Here's how the part is built. I have some questions about the finished solid (model axes, mm). Give positions to 0.01 mm unless a question says otherwise; leave off trailing zeros. Write each loop counter-clockwise with the first axis right and the second up, starting at its lowest first coordinate (ties: lowest second). Pieces come first, ordered by that corner, then holes. Notation, with made-up numbers: (-10.75, -7.5) - (10.25, -7.5) arc R20 cw to (10.25, 18.5) - close; hole circle Ø7 at (36, -18.5). An arc over 180 degrees is marked (long way). Use a Markdown table: item, result.
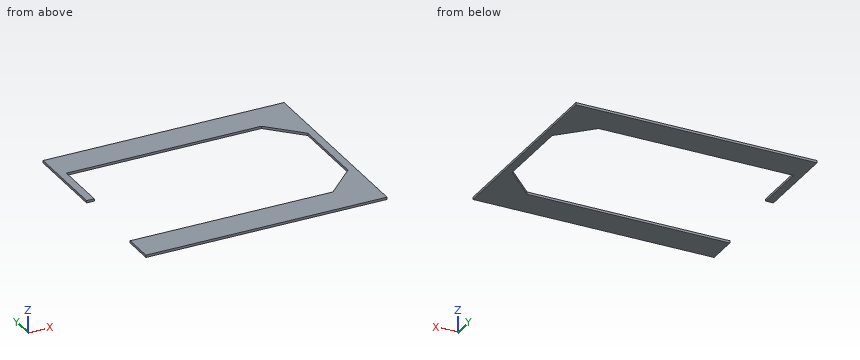
Autodesk Inventor part; units mm, degrees
ref_plane "YZ Plane" through (0, 0, 0) normal (1, 0, 0) x (0, 1, 0)
ref_plane "XZ Plane" through (0, 0, 0) normal (0, 1, 0) x (-1, 0, 0)
ref_plane "XY Plane" through (0, 0, 0) normal (0, 0, 1) x (1, 0, 0)
sketch "Эскиз1" plane through (0, 0, 0) normal (0, 0, 1) x (1, 0, 0)
  line L0 (0, 0) -> (-80.25, 0) construction
  line L1 (-80.25, 0) -> (-80.25, -18.086) construction
  line L2 (-80.25, -18.086) -> (0, -18.086) construction
  line L3 (0, -18.086) -> (0, 0) construction
  line L4 (-80.25, -18.086) -> (-80.25, -40.587) construction
  line L5 (-80.25, -18.086) -> (-57.749, -18.086) construction
  line L6 (-80.25, -40.587) -> (76.75, -40.587)
  line L7 (76.75, -40.587) -> (76.75, 90.413)
  line L8 (76.75, 90.413) -> (-80.25, 90.413)
  line L9 (-80.25, 90.413) -> (-80.25, -40.587)
  line L10 (-80.25, -40.587) -> (76.75, -40.587)
  line L11 (76.75, -40.587) -> (76.75, -20.587)
  line L12 (76.75, -20.587) -> (-80.25, -20.587)
  line L13 (-80.25, -20.587) -> (-80.25, -40.587)
  line L14 (76.75, 90.413) -> (-80.25, 90.413)
  line L15 (-80.25, 90.413) -> (-80.25, 70.413)
  line L16 (-80.25, 70.413) -> (76.75, 70.413)
  line L17 (76.75, 70.413) -> (76.75, 90.413)
  line L18 (-80.25, -40.587) -> (-75.25, -40.587)
  line L19 (-75.25, -40.587) -> (-75.25, 90.413)
  line L20 (-75.25, 90.413) -> (-80.25, 90.413)
  line L21 (-80.25, 90.413) -> (-80.25, -40.587)
  line L22 (76.75, -40.587) -> (71.75, -40.587)
  line L23 (71.75, -40.587) -> (71.75, 90.413)
  line L24 (71.75, 90.413) -> (76.75, 90.413)
  line L25 (76.75, 90.413) -> (76.75, -40.587)
  line L26 (76.75, -40.587) -> (41.75, -40.587)
  line L27 (41.75, -40.587) -> (41.75, -20.587)
  line L28 (41.75, -40.587) -> (61.75, -40.587) construction
  line L29 (76.75, 24.913) -> (-80.25, 24.913)
  line L30 (41.75, 90.413) -> (41.75, 70.413)
  line L31 (71.75, 70.413) -> (71.75, 50.413)
  line L32 (71.75, 50.413) -> (51.75, 70.413)
  line L33 (71.75, 50.413) -> (100.0343, 50.413) construction
  line L34 (71.75, -0.587) -> (51.75, -20.587)
  line L35 (-75.25, 24.913) -> (-80.25, 24.913)
  line L36 (-80.25, 24.913) -> (-80.25, 34.913)
  line L37 (-80.25, 34.913) -> (-75.25, 34.913)
  line L38 (-75.25, 34.913) -> (-75.25, 24.913)
  point P0 (-75.25, -20.587)
  point P1 (-75.25, 70.413)
  point P2 (71.75, -20.587)
  dimension "d0" = 80.25
  dimension "d1" = 18.086
  dimension "d2" = 22.501
  dimension "d3" = 90
  dimension "d4" = 157
  dimension "d5" = 131
  dimension "d6" = 157
  dimension "d7" = 20
  dimension "d8" = 157
  dimension "d9" = 20
  dimension "d10" = 5
  dimension "d11" = 131
  dimension "d12" = 5
  dimension "d13" = 131
  dimension "d16" = 35
  dimension "d17" = 20
  dimension "d18" = 90
  dimension "d19" = 20
  dimension "d20" = 135
  dimension "d21" = 10
extrude "Выдавливание1" add sketch "Эскиз1" along normal blind 1.5 contours L9 L12 L19 L6 | L19 L12 L27 L6 | L27 L12 L23 L6 | L23 L12 L7 L6 | L9 L16 L19 L37 | L23 L29 L7 L12 | L12 L34 L23 | L23 L16 L7 L29 | L9 L8 L19 L16 | L19 L8 L30 L16 | L32 L16 L23 | L30 L8 L23 L16 | L23 L8 L7 L16
sketch "Эскиз2" plane through (-80.25, -40.587, 0) normal (0, -1, 0) x (1, 0, 0)
  line L0 (132, 0) -> (0, 0)
  line L1 (157, 0) -> (0, 0)
  line L2 (0, 0) -> (157, 0)
  line L3 (157, 0) -> (78.5, 0)
  line L4 (78.5, 0) -> (78.5, -20)
  line L5 (78.5, -20) -> (73.5, -20)
  line L6 (73.5, -20) -> (49.6649, 0)
  line L7 (78.5, -20) -> (83.5, -20)
  line L8 (83.5, -20) -> (107.3351, 0)
  point P0 (80.25, 0)
  dimension "d22" = 20
  dimension "d24" = 5
  dimension "d25" = 140
properties part number "sensor board"
Item 1: Will this pin go through, and if not, where does the flat tip stop? pin 1 Ø3 at (x, y) = (-7, -20) entering from +Z.
Values:
| item | result |
|---|---|
| pin 1 | stops at z = 1.5 |
Item 2: If we section it at A-A, the plane y = 38.5: Write out the boundary of the cut face in (x, z), plus the area to 3 significant figures.
Values:
| item | result |
|---|---|
| outline | (-80.25, 0) - (-75.25, 0) - (-75.25, 1.5) - (-80.25, 1.5) - close; (71.75, 0) - (76.75, 0) - (76.75, 1.5) - (71.75, 1.5) - close |
| area | 15.0 mm2 |
Item 3: If we section it at C-C, the plane x = -13: Write out the boundary of the cut face in (y, z).
Values:
| item | result |
|---|---|
| outline | (-40.59, 0) - (-20.59, 0) - (-20.59, 1.5) - (-40.59, 1.5) - close; (70.41, 0) - (90.41, 0) - (90.41, 1.5) - (70.41, 1.5) - close |
Item 4: If we section it at D-D, the plane y = -16: Write out the boundary of the cut face in (x, z).
Values:
| item | result |
|---|---|
| outline | (56.34, 0) - (76.75, 0) - (76.75, 1.5) - (56.34, 1.5) - close |
Item 5: I need wall thicknesses on line 1 along Y through (x, z) = (3, 0.45); line 2 along X through (y, z) = (44, 0.95); line 3 along X through (y, z) = (5.5, 1.05). Which ranges of each line are inside material? Lowest first, please. Write a range as [from, to].
Values:
| item | result |
|---|---|
| line 1 | y = [-40.59, -20.59], [70.41, 90.41] |
| line 2 | x = [-80.25, -75.25], [71.75, 76.75] |
| line 3 | x = [71.75, 76.75] |
Item 6: If we section it at B-B, the plane z = 0.9: Write out the boundary of the cut face in (x, y), plus the area to 3 significant figures.
Values:
| item | result |
|---|---|
| outline | (-80.25, -40.59) - (76.75, -40.59) - (76.75, 90.41) - (-80.25, 90.41) - (-80.25, 34.91) - (-75.25, 34.91) - (-75.25, 70.41) - (51.75, 70.41) - (71.75, 50.41) - (71.75, -0.59) - (51.75, -20.59) - (-80.25, -20.59) - close |
| area | 7,310 mm2 |
